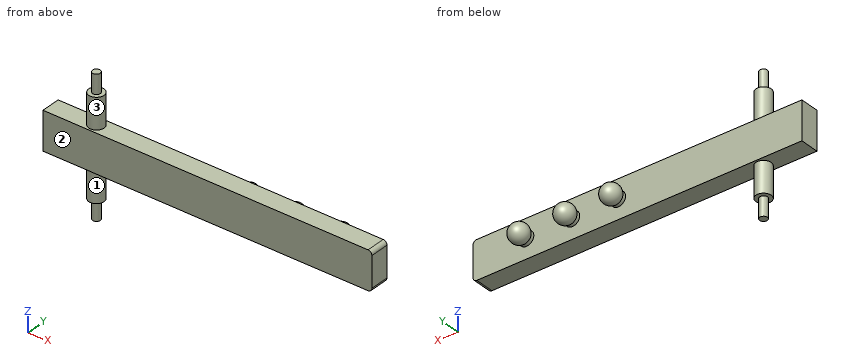
```python
from build123d import *

# Parameters (mm, degrees)
SKETCH_1_R              = 20
EXTRUDE_1_DEPTH         = 130
SKETCH_2_W              = 860
SKETCH_2_H              = 50
EXTRUDE_2_DEPTH         = 50
SKETCH_3_R              = 10
EXTRUDE_3_DEPTH         = 50
PATTERN_LINEAR_16_COUNT = 3
PATTERN_LINEAR_16_PITCH = 120
FILLET_1_R              = 10


with BuildPart() as part:
    # 草图1 → 凸台-拉伸1 (new body, symmetric)
    with BuildSketch(Plane.XY):
        Circle(SKETCH_1_R)
    extrude(amount=EXTRUDE_1_DEPTH, both=True)

    # 草图2 → 凸台-拉伸2 (add, symmetric)
    with BuildSketch(Plane.XY):
        with Locations((310, 0)):
            Rectangle(SKETCH_2_W, SKETCH_2_H)
    extrude(amount=EXTRUDE_2_DEPTH, both=True)

    # 草图3 → 凸台-拉伸3 (add)
    with BuildSketch(Plane.XY.offset(130)):
        Circle(SKETCH_3_R)
    extrude_3 = extrude(amount=EXTRUDE_3_DEPTH)

    # 镜向1: 凸台-拉伸3 across plane
    add(extrude_3.mirror(Plane.XY))

    # 草图6 → 旋转3 (revolve)
    with BuildSketch(Plane.XY):
        with BuildLine():
            Line((360, 75), (360, 50))
            Line((360, 50), (360, 25))
            Line((360, 25), (378.993679067, 25))
            Line((378.993679067, 25), (378.993679067, 33.744534596))
            ThreePointArc((378.993679067, 33.744534596), (382.708881909, 60.454983618), (360, 75))
        make_face()
    revolve_3 = revolve(axis=Axis((360, 25, 0), (0, 1, 0)))

    # 阵列(线性)16: 旋转3 ×3
    with Locations(*[(i * PATTERN_LINEAR_16_PITCH, 0, 0) for i in range(1, PATTERN_LINEAR_16_COUNT)]):
        add(revolve_3)

    # 圆角1
    fillet_1_edges = [part.edges().sort_by_distance(p)[0] for p in [
        (740, 0, -50),
        (740, 0, 50),
    ]]
    fillet(fillet_1_edges, radius=FILLET_1_R)


solid = part.part
```
Input: part model. Units: mm. Frame: model coordinates. Face numbers are marked on the shaded views. A direction names the side the tool comes from. Coordinates: 2 decimals unless noted, no trailing zeros. Loops run counter-clockwise (first coordinate to the right, second up) from the corner with the lowest first, then second, coordinate; pieces in that order, holes last. Notation, with made-up numbers: (20.25, -7.5) -> (56.25, -7.5) arc R17 ccw to (56.25, 4.5) -> close; hole circle Ø11 at (35.25, 20.5). An arc over 180 degrees is marked (long way). Use a Markdown table: item, result.
1) Access query for the marked faces 1, 2 and 3. Directions: +Z, -Z, +X, -X, +Y, -Y. A direction counts if a zero-diameter tool reaches every point of the face in a straight line with its end or side. Return the directions, or none.
Results found:
| item | result |
|---|---|
| face 1 | -Z |
| face 2 | +Z, -Z, +X, -X, -Y |
| face 3 | +Z |
2) Cut plane B-B (x = 600). Return the cut outline in (y, z), then the cut area to 3 significant figures.
Results found:
| item | result |
|---|---|
| outline | (-25, -50) -> (25, -50) -> (25, -18.99) -> (33.74, -18.99) arc R25 ccw (long way) to (33.74, 18.99) -> (25, 18.99) -> (25, 50) -> (-25, 50) -> close |
| area | 7,070 mm2 |
3) Material intervals for line 1 along Y through (x, z) = (75.5, -17); line 2 along X through (y, z) = (62, -1); line 3 along Z through (x, y) = (580, 23.5), sorted ascending. Write a range as from..to.
Results found:
| item | result |
|---|---|
| line 1 | y = -25..25 |
| line 2 | x = 338.09..381.91, 458.09..501.91, 578.09..621.91 |
| line 3 | z = -50..50 |
4) Cut plane C-C (y = 0). Return the cut outline in (x, z), then the cut area to 3 significant figures.
Results found:
| item | result |
|---|---|
| outline | (-120, -50) -> (-20, -50) -> (-20, -130) -> (-10, -130) -> (-10, -180) -> (10, -180) -> (10, -130) -> (20, -130) -> (20, -50) -> (730, -50) arc R10 ccw to (740, -40) -> (740, 40) arc R10 ccw to (730, 50) -> (20, 50) -> (20, 130) -> (10, 130) -> (10, 180) -> (-10, 180) -> (-10, 130) -> (-20, 130) -> (-20, 50) -> (-120, 50) -> close |
| area | 94,400 mm2 |
5) Cut plane A-A (z = 0). Return the cut outline in (x, y), then the cut area to 3 significant figures.
Results found:
| item | result |
|---|---|
| outline | (-120, -25) -> (740, -25) -> (740, 25) -> (618.99, 25) -> (618.99, 33.74) arc R25 ccw (long way) to (581.01, 33.74) -> (581.01, 25) -> (498.99, 25) -> (498.99, 33.74) arc R25 ccw (long way) to (461.01, 33.74) -> (461.01, 25) -> (378.99, 25) -> (378.99, 33.74) arc R25 ccw (long way) to (341.01, 33.74) -> (341.01, 25) -> (-120, 25) -> close |
| area | 49,200 mm2 |
6) Cut plane D-D (x = 0). Return the cut outline in (y, z), then the cut area to 3 significant figures.
Results found:
| item | result |
|---|---|
| outline | (-25, -50) -> (-20, -50) -> (-20, -130) -> (-10, -130) -> (-10, -180) -> (10, -180) -> (10, -130) -> (20, -130) -> (20, -50) -> (25, -50) -> (25, 50) -> (20, 50) -> (20, 130) -> (10, 130) -> (10, 180) -> (-10, 180) -> (-10, 130) -> (-20, 130) -> (-20, 50) -> (-25, 50) -> close |
| area | 13,400 mm2 |
7) Contact query for flat-ended pins moving along their axis: pin 1 (15 mm diameter, centred on x = 451.5, y = 4, fed in from -Z); pin 2 (1.5 mm diameter, centred on x = 108.5, y = 18.5, fed in from +Z); pin 3 (5 mm diameter, centred on y = 15, z = -76, fed in from +X). Output: stop coordinate, or through.
Results found:
| item | result |
|---|---|
| pin 1 | stops at z = -50 |
| pin 2 | stops at z = 50 |
| pin 3 | stops at x = 15.61 |
